Design review of the part built by this model. Coordinates are the model's own, in mm. A direction names the side the tool comes from. Round coordinates to 2 decimals unless told otherwise and drop trailing zeros. Order: outer loops, then holes, each group sorted by start corner. A loop starts at its lowest first (then second) coordinate and runs counter-clockwise, first axis right, second up. Notation, with made-up numbers: (26, 29) - (51, 29) arc R8 ccw to (51, 34) - close; hole circle Ø2 at (-8, 0). An arc over 180 degrees is marked (long way). Use CSV: the item, a comma, the result in double quotes.
from build123d import *

# Parameters (mm, degrees)
CROQUIS2_OUTSIDE_W    = 43.94
CROQUIS2_OUTSIDE_H    = 43.94
CORTAR_EXTRUIR1_DEPTH = 25


with BuildPart() as part:
    # Croquis1 → Revolución1 (revolve)
    with BuildSketch(Plane.XY):
        Polygon((8.025, 24), (8.025, -18), (9.525, -18), (11.11, 0), (15, 0), (15, 6), (11.11, 6), (9.525, 24), align=None)
    revolve(axis=Axis((0, 30.334405112, 0), (0, -1, 0)))

    # Croquis2 outside → Cortar-Extruir1 (cut, through all)
    with BuildSketch(Plane(origin=(0, 6, 0), x_dir=(1, 0, 0), z_dir=(0, 1, 0))):
        Rectangle(CROQUIS2_OUTSIDE_W, CROQUIS2_OUTSIDE_H)
        Polygon((15, 0), (7.5, 12.990381057), (-7.5, 12.990381057), (-15, 0), (-7.5, -12.990381057), (7.5, -12.990381057), align=None, mode=Mode.SUBTRACT)
    extrude(amount=-CORTAR_EXTRUIR1_DEPTH, mode=Mode.SUBTRACT)


solid = part.part
1) For faces 1 (the face through (3, 6, 11)), 2 (the face through (-3, 0, 11)), 3 (the face through (11.198, 3.042, 6.586)), list the 3-axis set-ups (+Z, -Z, +X, -X, +Y, -Y) from which the entire face can be reached by the end or side of a thin tool; tool diameter is ignored.
Data:
face 1,"+Y"
face 2,"-Y"
face 3,"+Z, +X, +Y, -Y"
2) We need section C-C (y = 18.5). Give the boundary of the cut face in (x, z) (3 decimals).
Data:
outline,"circle Ø20.019 at (0, 0); hole circle Ø16.05 at (0, 0)"
3) Insertion check: pin 1 Ø5 at (x, y) = (-6, 16) entering from +Z; pin 2 Ø8 at (x, y) = (0, 10.5) entering from +Z; pin 3 Ø10 at (y, z) = (17, 3) entering from -X. Each pin has a flat end and moves straight along its axis. Give the tip position at first contact, or say it passes through.
Data:
pin 1,"stops at z = 9.64"
pin 2,"stops at z = 11.07"
pin 3,"stops at x = -10.51"
4) We need section D-D (y = 9). Give the boundary of the cut face in (x, z) (3 decimals).
Data:
outline,"circle Ø21.692 at (0, 0); hole circle Ø16.05 at (0, 0)"
5) The part is to be moulded in two halves that separate along Z. For faces 4 (the face through (-8.18, 15.13, -6.27)), 5 (the face through (11.302, 3.042, -6.404)), 6 (the face through (0, 3, 12.99)), 7 (the face through (-6.37, 2.71, -4.88)), say which applies: +Z half, -Z half, draft (parallel to the pull), parting line (faces both ways), or undercut.
Data:
face 4,"parting line"
face 5,"-Z half"
face 6,"+Z half"
face 7,"undercut"
6) We need section A-A (y = 0.5). Give the boundary of the cut face in (x, z) (3 decimals), then the cut area to 3 significant figures.
Data:
outline,"(-15, 0) - (-7.5, -12.99) - (7.5, -12.99) - (15, 0) - (7.5, 12.99) - (-7.5, 12.99) - close; hole circle Ø16.05 at (0, 0)"
area,"382 mm2"
7) We need section B-B (x = 0). Give the boundary of the cut face in (y, z) (3 decimals), then the cut area to 3 significant figures.
Data:
outline,"(-18, -9.525) - (0, -11.11) - (0, -12.99) - (6, -12.99) - (6, -11.11) - (24, -9.525) - (24, -8.025) - (-18, -8.025) - close; (-18, 8.025) - (24, 8.025) - (24, 9.525) - (6, 11.11) - (6, 12.99) - (0, 12.99) - (0, 11.11) - (-18, 9.525) - close"
area,"225 mm2"
8) To check wall thickness, follow L1, parallel to Y at x = -9, z = 8.5; L2, parallel to Z at x = 7.25, y = 3; L3, parallel to Z at x = 0, y = 8 (3 decimals). State the ranges of each line that lie inside material, in increasing order. Write a range as from..to.
Data:
L1,"y = 0..6"
L2,"z = -12.99..-3.44, 3.44..12.99"
L3,"z = -10.934..-8.025, 8.025..10.934"
